Autodesk Inventor part; units mm, degrees
ref_plane "Work Plane1" through (-16.5, 0, 0) normal (1, 0, 0) x (0, 0, -1)
ref_plane "YZ Plane" through (0, 0, 0) normal (1, 0, 0) x (0, 1, 0)
ref_plane "XZ Plane" through (0, 0, 0) normal (0, 1, 0) x (-1, 0, 0)
sketch "Sketch1" plane through (0, 0, 0) normal (0, 1, 0) x (-1, 0, 0)
  line L0 (0, 0) -> (33, 0)
  line L1 (33, 0) -> (33, -10)
  line L2 (33, -10) -> (0, -10)
  line L3 (0, -10) -> (0, 0)
  dimension "d0" = 33
  dimension "d1" = 10
extrude "Extrusion1" add sketch "Sketch1" along normal blind 4
sketch "Sketch2" plane through (0, 4, 0) normal (0, 1, 0) x (1, 0, 0)
  circle A0 centre (-5.343, 5) radius 1.8
  point P0 (0, 0)
  dimension "d9" = 3.6
extrude "Extrusion2" cut sketch "Sketch2" against normal blind 4
ref_plane "Work Plane1" through (-16.5, 0, 0) normal (1, 0, 0) x (0, 0, -1)
mirror "Mirror1" about plane through (-16.5, 0, 0) normal (1, 0, 0) of "Extrusion2"
fillet "Fillet1" radius 3 4 edges at (-33, 2, 0) (-33, 2, -10) (0, 2, 0) (0, 2, -10)
properties part number "9 peristaltic pump clamp"
Part model, mm, in its own coordinate system. Coordinates: 2 decimals unless noted, no trailing zeros. Write each loop counter-clockwise with the first axis right and the second up, starting at its lowest first coordinate (ties: lowest second). Pieces come first, ordered by that corner, then holes.
Item 1: Slice it at C-C (x = -6). Write the cut outline in (y, z), and give its area (3 significant figures).
Item 2: Probe line 1 (X direction, y = 2.95, z = -5); line 2 (X direction, y = 0.25, z = -6); line 3 (Z direction, x = -27, y = 2.35). List the from-to ranges inside material, lowest first.
Item 3: Slice it at B-B (y = 2.3). Write the cut outline in (x, z).
Item 4: Slice it at A-A (z = -5). Write the cut outline in (x, y).
Item 5: Slice it at D-D (z = -0.75). Write the cut outline in (x, y).
Item 6: Mould opens along Z. For faces 1 (the face through (-0.86, 2.03, -9.1)), 2 (the face through (-5.733, 2.028, -3.243)), 3 (the face through (-33, 2, -5)) say: released by +Z, released by -Z, zero draft, split by the parting line, or undercut.
Item 7: Pin check, flat tips, straight feed: pin 1 (2 mm diameter, centred on x = -5.343, z = -5, fed in from -Y) (3 decimals); pin 2 (2 mm diameter, centred on y = 3, z = -2.5, fed in from +X). Stop position of each tip, or through.
Results found:
1. outline: (0, -10) - (4, -10) - (4, -6.68) - (0, -6.68) - close; (0, -3.32) - (4, -3.32) - (4, 0) - (0, 0) - close
1. area: 26.6 mm2
2. line 1: x = -33 to -29.46, -25.86 to -7.14, -3.54 to 0
2. line 2: x = -33 to -29.15, -26.16 to -6.84, -3.85 to 0
2. line 3: z = -10 to -6.68, -3.32 to 0
3. outline: (-33, -7) arc R3 ccw to (-30, -10) - (-3, -10) arc R3 ccw to (0, -7) - (0, -3) arc R3 ccw to (-3, 0) - (-30, 0) arc R3 ccw to (-33, -3) - close; hole circle Ø3.6 at (-27.66, -5); hole circle Ø3.6 at (-5.34, -5)
4. outline: (-33, 0) - (-29.46, 0) - (-29.46, 4) - (-33, 4) - close; (-25.86, 0) - (-7.14, 0) - (-7.14, 4) - (-25.86, 4) - close; (-3.54, 0) - (0, 0) - (0, 4) - (-3.54, 4) - close
5. outline: (-31.98, 0) - (-1.02, 0) - (-1.02, 4) - (-31.98, 4) - close
6. face 1: released by -Z
6. face 2: undercut
6. face 3: zero draft
7. pin 1: passes through
7. pin 2: stops at x = 0
